```python
from build123d import *

# Parameters (mm, degrees)
F0_R     = 40
F1_DEPTH = 2
F3_DEPTH = 25


with BuildPart() as f1:
    # F0 (on Top) → F1 (new body)
    with BuildSketch(Plane.XY):
        Circle(F0_R)
    extrude(amount=F1_DEPTH)

    # F2 (on face) → F3 (cut)
    with BuildSketch(Plane.XY.offset(2)):
        with BuildLine():
            ThreePointArc((-25.405787, 6.224418), (-9.867491, 0.583944), (0, 13.846154))
            ThreePointArc((0, 13.846154), (-17.824817, 27.108364), (-25.405787, 6.224418))
        make_face()
        with BuildLine():
            ThreePointArc((25.405787, 6.224418), (9.867491, 0.583944), (0, 13.846154))
            ThreePointArc((0, 13.846154), (-9.867491, 0.583944), (-25.405787, 6.224418))
            Line((-25.405787, 6.224418), (0, -32.307692))
            Line((0, -32.307692), (25.405787, 6.224418))
        make_face()
        with BuildLine():
            ThreePointArc((27.692308, 13.846154), (13.846154, 27.692308), (0, 13.846154))
            ThreePointArc((0, 13.846154), (9.867491, 0.583944), (25.405787, 6.224418))
            ThreePointArc((25.405787, 6.224418), (27.108364, 9.867491), (27.692308, 13.846154))
        make_face()
    extrude(amount=-F3_DEPTH, mode=Mode.SUBTRACT)


solid = f1.part
```
Geometry check sheet. Reference: the model listing, model coordinates, mm. A direction names the side the tool comes from. Give positions to 0.01 mm unless a question says otherwise; leave off trailing zeros. Write each loop counter-clockwise with the first axis right and the second up, starting at its lowest first coordinate (ties: lowest second). Pieces come first, ordered by that corner, then holes.
1) Section check D-D, the plane y = 0. Record the boundary of the cut face in (x, z), and give its area (3 significant figures).
2) Section check C-C, the plane y = 22.5. Record the boundary of the cut face in (x, z).
3) Section check A-A, the plane x = -18. Record the boundary of the cut face in (y, z).
4) Access from +Z, -Z, +X, -X, +Y, -Y to the whole of each face (thin tool, end or side, straight path). Record for faces 4 (the flat face through (17, -8, 0)), 5 (the flat face through (12.525, -13.311, 1.014)).
5) Section check B-B, the plane z = 0.5. Record the boundary of the cut face in (x, y).
6) Release check for a two-part mould opening along Y. For faces 1 (the cylindrical face through (-17.5, 27.2, 1)), 2 (the cylindrical face through (-8.67, -39.05, 0.99)), 3 (the flat face through (17, -8, 2)) record: pulls with the +Y half, pulls with the -Y half, needs draft (parallel to the pull), parting line crosses it, or undercut.
7) Material ranges on L1, parallel to X at y = 16, z = 0.25; L2, parallel to X at y = 24.5, z = 0.35; L3, parallel to Y at x = 6, z = 1.3, recorded low to high.
Computed:
1. outline: (-40, 0) - (-21.3, 0) - (-21.3, 2) - (-40, 2) - close; (21.3, 0) - (40, 0) - (40, 2) - (21.3, 2) - close
1. area: 74.8 mm2
2. outline: (-33.07, 0) - (-24.65, 0) - (-24.65, 2) - (-33.07, 2) - close; (-3.04, 0) - (3.04, 0) - (3.04, 2) - (-3.04, 2) - close; (24.65, 0) - (33.07, 0) - (33.07, 2) - (24.65, 2) - close
3. outline: (-35.72, 0) - (-5.01, 0) - (-5.01, 2) - (-35.72, 2) - close; (27.05, 0) - (35.72, 0) - (35.72, 2) - (27.05, 2) - close
4. face 4: -Z, +X, -X, +Y, -Y
4. face 5: +Z, -Z
5. outline: circle Ø80 at (0, 0); hole (-25.41, 6.22) - (0, -32.31) - (25.41, 6.22) arc R13.85 ccw to (27.69, 13.85) arc R13.85 ccw to (0, 13.85) arc R13.85 ccw (long way) to start
6. face 1: undercut
6. face 2: parting line crosses it
6. face 3: needs draft
7. L1: x = -36.66 to -27.52, -0.17 to 0.17, 27.52 to 36.66
7. L2: x = -31.62 to -22.69, -5 to 5, 22.69 to 31.62
7. L3: y = -39.55 to -23.21, 25.25 to 39.55
